Here's how the part is built. I have some questions about the finished solid (model axes, mm). A direction names the side the tool comes from. Give positions to 0.01 mm unless a question says otherwise; leave off trailing zeros. Loops run counter-clockwise (first coordinate to the right, second up) from the corner with the lowest first, then second, coordinate; pieces in that order, holes last. Notation, with made-up numbers: M 86,52 L 118,52 A20 cw 118,78 Z; hole C 13.25,-2.5 d8. An arc over 180 degrees is marked long. Answer as CSV lines item,"result". Start each with the question number.
Item 1: I want a section at D-D on y = -44.5. List the corners of the cut face in (x, z) for me.
Item 2: If I drill on line 1 along Y through (x, z) = (-3.75, -6.75); line 2 along X through (y, z) = (-72.6, -11); line 3 along Z through (x, y) = (2.5, 18.5), over which ranges is the centre line in solid material (lowest first)? Write a range as from..to.
Item 3: If we mould it in two halves opening along Z, with no side actions, what happens to faces 1 (the flat face through (0, 74, -15)), 2 (the flat face through (0, 76.2, -5)), 3 (the cylindrical face through (-0.51, -73.67, -9.38))? For each: released by +Z, released by -Z, zero draft, split by the parting line, or undercut.
Item 4: I want a section at B-B on z = -19. List the corners of the cut face in (x, y) for me, plus the area to 3 significant figures.
Item 5: I want a section at A-A on z = -11. List the corners of the cut face in (x, y) for me.
Item 6: Will these pins go through, and if not, where does the flat tip stop? P1, Ø5.5, axis at x = -1, y = 14, coming from the -Z side; P2, Ø3, axis at x = -2, y = 73.5, coming from the -Z side.
Item 7: For faces 4 (the flat face through (0, 1, -5)), 5 (the flat face through (5.5, 0, -4)), which set-ups out of +Z, -Z, +X, -X, +Y, -Y let a thin tool reach every point of the face, with its end or its side?
Item 8: I want a section at C-C on x = 0. List the corners of the cut face in (y, z) for me.
from build123d import *

# Parameters (mm, degrees)
SKETCH1_W           = 11
SKETCH1_H           = 10
BOSS_EXTRUDE1_DEPTH = 76.2
SKETCH3_W           = 11
SKETCH3_H           = 20
SKETCH3_R           = 1.7
BOSS_EXTRUDE3_DEPTH = 4
BOSS_EXTRUDE4_START = -5
SKETCH4_W           = 11
SKETCH4_H           = 28
SKETCH4_R           = 1.7
BOSS_EXTRUDE4_DEPTH = 5
FILLET1_R           = 1.5


with BuildPart() as part:
    # Sketch1 → Boss-Extrude1 (new, symmetric)
    with BuildSketch(Plane(origin=(0, 0, 0), x_dir=(1, 0, 0), z_dir=(0, 1, 0))):
        Rectangle(SKETCH1_W, SKETCH1_H)
    extrude(amount=BOSS_EXTRUDE1_DEPTH, both=True)

    # Sketch3 → Boss-Extrude3 (add)
    with BuildSketch(Plane(origin=(0, 76.2, 0), x_dir=(1, 0, 0), z_dir=(0, 1, 0))):
        with Locations((0, 5)):
            Rectangle(SKETCH3_W, SKETCH3_H)
        with Locations(Location((0, 11, 0), (0, 0, 270))):
            Circle(SKETCH3_R, mode=Mode.SUBTRACT)
    extrude(amount=-BOSS_EXTRUDE3_DEPTH)

    # Sketch4 → Boss-Extrude4 (add)
    with BuildSketch(Plane.XZ.offset(76.2).offset(BOSS_EXTRUDE4_START)):
        with Locations((0, -9)):
            Rectangle(SKETCH4_W, SKETCH4_H)
        with Locations(Location((0, -11, 0), (0, 0, 90))):
            Circle(SKETCH4_R, mode=Mode.SUBTRACT)
        with Locations(Location((0, -19, 0), (0, 0, 270))):
            Circle(SKETCH4_R, mode=Mode.SUBTRACT)
    extrude(amount=BOSS_EXTRUDE4_DEPTH)

    # Fillet1
    fillet1_edges = [part.edges().sort_by_distance(p)[0] for p in [
        (0, 72.2, -5),
        (0, -71.2, -5),
    ]]
    fillet(fillet1_edges, radius=FILLET1_R)


solid = part.part
Result:
1,outline,"M -5.5,-5 L 5.5,-5 L 5.5,5 L -5.5,5 Z"
2,line 1,"-76.2..-71.2, 72.2..76.2"
2,line 2,"-5.5..-1.7, 1.7..5.5"
2,line 3,"-5..5"
3,face 1,"released by -Z"
3,face 2,"zero draft"
3,face 3,"undercut"
4,outline,"M -5.5,-76.2 L -1.7,-76.2 L -1.7,-71.2 L -5.5,-71.2 Z; M 1.7,-76.2 L 5.5,-76.2 L 5.5,-71.2 L 1.7,-71.2 Z"
4,area,"38.0 mm^2"
5,outline,"M -5.5,-76.2 L -1.7,-76.2 L -1.7,-71.2 L -5.5,-71.2 Z; M -5.5,72.2 L -1.7,72.2 L -1.7,76.2 L -5.5,76.2 Z; M 1.7,-76.2 L 5.5,-76.2 L 5.5,-71.2 L 1.7,-71.2 Z; M 1.7,72.2 L 5.5,72.2 L 5.5,76.2 L 1.7,76.2 Z"
6,P1,"z = -5"
6,P2,"z = -15"
7,face 4,"-Z, +X, -X"
7,face 5,"+Z, -Z, +X, +Y, -Y"
8,outline,"M -76.2,-23 L -71.2,-23 L -71.2,-20.7 L -76.2,-20.7 Z; M -76.2,-17.3 L -71.2,-17.3 L -71.2,-12.7 L -76.2,-12.7 Z; M -76.2,-9.3 L -71.2,-9.3 L -71.2,-6.5 A1.5 cw -69.7,-5 L 70.7,-5 A1.5 cw 72.2,-6.5 L 72.2,-9.3 L 76.2,-9.3 L 76.2,5 L -76.2,5 Z; M 72.2,-15 L 76.2,-15 L 76.2,-12.7 L 72.2,-12.7 Z"
